Read the model definition and answer for the solid it produces. Units are mm, in the model's axes. Face numbers are marked on the shaded views. A direction names the side the tool comes from. Round coordinates to 2 decimals unless told otherwise and drop trailing zeros. Order: outer loops, then holes, each group sorted by start corner. A loop starts at its lowest first (then second) coordinate and runs counter-clockwise, first axis right, second up. Notation, with made-up numbers: (28.25, 88) -> (75.25, 88) arc R31 cw to (75.25, 115) -> close; hole circle Ø1 at (22.5, -32). An arc over 180 degrees is marked (long way). Answer as a JSON object with one key per item and string values. Group by question number.
Item 1: Section B-B, the plane z = -25 is taken. Write down the section's boundary in (x, y).
Item 2: The mould has two halves that part along Z. Classify the marked faces 1, 2, 3 and 4: pulls with the +Z half, pulls with the -Z half, needs draft (parallel to the pull), parting line crosses it, or undercut.
Item 3: Section D-D, the plane z = 23.5 is taken. Write down the section's boundary in (x, y), plus the area to 3 significant figures.
Item 4: Consider probe 1 along Y at (x, z) = (-16.5, -25); probe 2 along Z at (x, y) = (-13.25, -90); probe 3 along X at (y, z) = (-23.5, -25). Determine where each line is inside the solid, lowest interval first. Write a range as from..to.
Item 5: Section A-A, the plane y = -51.5 is taken. Write down the section's boundary in (x, z), plus the area to 3 significant figures.
Item 6: For the marked faces 5, 6, 7, 8 and 9, determine the directions among +Z, -Z, +X, -X, +Y, -Y from which every point of the face is accessible in a straight line to the end or side of a thin tool.
Item 7: Given P1, Ø5, axis at x = -4, z = 25, coming from the -Y side; P2, Ø5, axis at y = -49, z = 2.5, coming from the -X side; P3, Ø5, axis at x = -7, y = 18, coming from the -Z side; P4, Ø7, axis at y = -90, z = 25, coming from the +X side (1 decimal), each flat-ended and moving along its own axis, determine where each tip first touches the part or whether it passes through.
Item 8: Section C-C, the plane y = 15 is taken. Write down the section's boundary in (x, z).
from build123d import *

# Parameters (mm, degrees)
Y_KSEKLIK_EKSTR_ZYON1_DEPTH = 45
Y_KSEKLIK_EKSTR_ZYON2_DEPTH = 75
IZIM3_R                     = 10
KES_EKSTR_ZYON1_DEPTH       = 75
IZIM4_R                     = 6
KES_EKSTR_ZYON2_DEPTH       = 11
Y_KSEKLIK_EKSTR_ZYON3_DEPTH = 6
Y_KSEKLIK_EKSTR_ZYON4_DEPTH = 3


with BuildPart() as part:
    # Çizim1 → Yükseklik-Ekstrüzyon1 (new body, symmetric)
    with BuildSketch(Plane.XY):
        Polygon((0, 0), (0, -75), (-10, -75), (-10, -105), (-20, -105), (-20, -65), (-10, -65), (-10, -10), (-20, -10), (-20, 30), (-10, 30), (-10, 0), align=None)
    extrude(amount=Y_KSEKLIK_EKSTR_ZYON1_DEPTH, both=True)

    # Çizim2 → Yükseklik-Ekstrüzyon2 (add)
    with BuildSketch(Plane(origin=(0, 0, 0), x_dir=(1, 0, 0), z_dir=(0, 1, 0))):
        with BuildLine():
            Line((0, 45), (35, 45))
            ThreePointArc((35, 45), (55, 25), (35, 5))
            Line((35, 5), (0, 5))
            Line((0, 5), (0, 45))
        make_face()
    extrude(amount=-Y_KSEKLIK_EKSTR_ZYON2_DEPTH)

    # Çizim3 → Kes-Ekstrüzyon1 (cut)
    with BuildSketch(Plane(origin=(0, 0, 0), x_dir=(1, 0, 0), z_dir=(0, 1, 0))):
        with Locations((35, 25)):
            Circle(IZIM3_R)
    extrude(amount=-KES_EKSTR_ZYON1_DEPTH, mode=Mode.SUBTRACT)

    # Çizim4 → Kes-Ekstrüzyon2 (cut, through all)
    with BuildSketch(Plane(origin=(-10, 0, 0), x_dir=(0, 0, -1), z_dir=(1, 0, 0))):
        with Locations((-25, 15)):
            Circle(IZIM4_R)
        with Locations((25, 15)):
            Circle(IZIM4_R)
    kes_ekstr_zyon2 = extrude(amount=-KES_EKSTR_ZYON2_DEPTH, mode=Mode.SUBTRACT)

    # Aynalama1: Kes-Ekstrüzyon2 across plane
    add(kes_ekstr_zyon2.mirror(Plane.ZX.offset(-37.5)), mode=Mode.SUBTRACT)

    # Çizim5 → Yükseklik-Ekstrüzyon3 (add)
    with BuildSketch(Plane.XY.offset(8)):
        Polygon((-10, 30), (0, 0), (-10, 0), align=None)
    y_kseklik_ekstr_zyon3 = extrude(amount=-Y_KSEKLIK_EKSTR_ZYON3_DEPTH)

    # Aynalama2: Yükseklik-Ekstrüzyon3 across plane
    add(y_kseklik_ekstr_zyon3.mirror(Plane.ZX.offset(-37.5)))

    # Çizim6 → Yükseklik-Ekstrüzyon4 (add, symmetric)
    with BuildSketch(Plane(origin=(0, -37.5, 0), x_dir=(1, 0, 0), z_dir=(0, 1, 0))):
        Polygon((0, 9.626666966), (45, 9.626666966), (0, -45), align=None)
    extrude(amount=Y_KSEKLIK_EKSTR_ZYON4_DEPTH, both=True)


solid = part.part
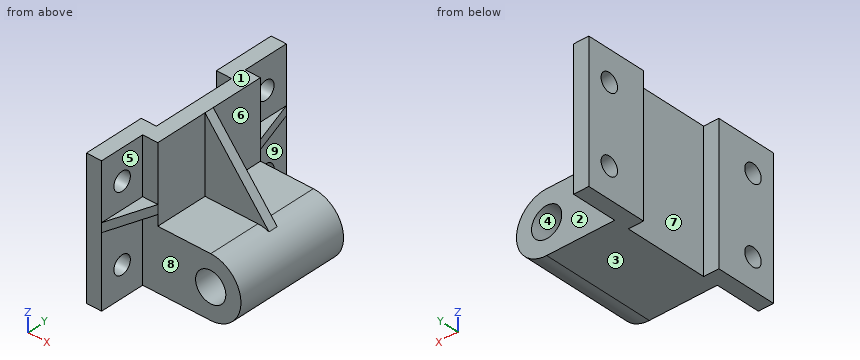
Values found:
{
 "1": {"outline": "(-20, -105) -> (-10, -105) -> (-10, -96) -> (-20, -96) -> close; (-20, -84) -> (-10, -84) -> (-10, -75) -> (25, -75) -> (25, 0) -> (-10, 0) -> (-10, 9) -> (-20, 9) -> (-20, -10) -> (-10, -10) -> (-10, -65) -> (-20, -65) -> close; (-20, 21) -> (-10, 21) -> (-10, 30) -> (-20, 30) -> close; (45, -75) -> (55, -75) -> (55, 0) -> (45, 0) -> close"},
 "2": {"face 1": "pulls with the +Z half", "face 2": "needs draft", "face 3": "pulls with the -Z half", "face 4": "undercut"},
 "3": {"outline": "(-20, -105) -> (-10, -105) -> (-10, -95.81) -> (-20, -95.81) -> close; (-20, -84.19) -> (-10, -84.19) -> (-10, -75) -> (0, -75) -> (0, -40.5) -> (17.71, -40.5) -> (17.71, -34.5) -> (0, -34.5) -> (0, 0) -> (-10, 0) -> (-10, 9.19) -> (-20, 9.19) -> (-20, -10) -> (-10, -10) -> (-10, -65) -> (-20, -65) -> close; (-20, 20.81) -> (-10, 20.81) -> (-10, 30) -> (-20, 30) -> close", "area": "1,420 mm2"},
 "4": {"probe 1": "-105..-96, -84..-65, -10..9, 21..30", "probe 2": "-45..-31, -19..19, 31..45", "probe 3": "-10..25, 45..55"},
 "5": {"outline": "(-10, -45) -> (35, -45) arc R20 ccw to (35, -5) -> (0, -5) -> (0, 45) -> (-10, 45) -> close; hole circle Ø20 at (35, -25)", "area": "2,610 mm2"},
 "6": {"face 5": "+Z, +X, -Y", "face 6": "+Z, +X, +Y", "face 7": "+Z, -Z, -X", "face 8": "-Z, +X, -Y", "face 9": "-Z, +X, +Y"},
 "7": {"P1": "y = -75", "P2": "x = -10", "P3": "z = 2", "P4": "through"},
 "8": {"outline": "(-20, -45) -> (-10, -45) -> (-10, -31) -> (-20, -31) -> close; (-20, -19) -> (-10, -19) -> (-10, 2) -> (-5, 2) -> (-5, 8) -> (-10, 8) -> (-10, 19) -> (-20, 19) -> close; (-20, 31) -> (-10, 31) -> (-10, 45) -> (-20, 45) -> close"}
}
